Design review of the part built by this model. Coordinates are the model's own, in mm. A direction names the side the tool comes from. Coordinates: 2 decimals unless noted, no trailing zeros. Loops run counter-clockwise (first coordinate to the right, second up) from the corner with the lowest first, then second, coordinate; pieces in that order, holes last. Notation, with made-up numbers: (16.25, -19.5) -> (73.25, -19.5) arc R23 cw to (73.25, 5.5) -> close; hole circle Ø11 at (-10.75, -19). An arc over 180 degrees is marked (long way). Use a Markdown table: item, result. Add a question column.
Q1. Clearance check with flat-ended pins moving along their axes: pin 1 Ø0.9 at (y, z) = (22, 2) entering from -X; pin 2 Ø1.5 at (x, z) = (26.5, 2) entering from -Y; pin 3 Ø1.5 at (x, z) = (25.5, 2) entering from +Y. State where each tip first meets the part, or that it passes through.
Q2. For faces 1 (the face through (21.82, -22, 2)), 2 (the face through (-21.82, 22, 2)), 3 (the face through (21.82, 21, 2)), 4 (the face through (-27, -20, 2)), list the 3-axis set-ups (+Z, -Z, +X, -X, +Y, -Y) from which the entire face can be reached by the end or side of a thin tool; tool diameter is ignored.
Q3. Take a section at B-B on x = 22.5. Write out the cut boundary in (y, z).
Q4. Take a section at A-A on z = 1.2. Write out the cut boundary in (x, y).
Q5. For probe 1 along Y at (x, z) = (27, 2.25); probe 2 along X at (y, z) = (-21, 2.65), list the stretches that pass through material, from the lowest coordinate up.
Solid Edge part; units mm, degrees
sketch "Sketch1" plane through (0, 0, 0) normal (0, 0, 1) x (1, 0, 0)
  line L0 (-31.82, -23) -> (31.82, -23)
  line L1 (31.82, -23) -> (31.82, 23)
  line L2 (31.82, 23) -> (-31.82, 23)
  line L3 (-31.82, 23) -> (-31.82, -23)
  dimension "D1" = 31.82
  dimension "D2" = 31.82
extrude "Ajout_matière_1" add sketch "Sketch1" along normal blind 3
sketch "Sketch2" plane through (0, 0, 3) normal (0, 0, 1) x (1, 0, 0)
  line L0 (-31.82, 23) -> (-21.82, 23)
  line L1 (-21.82, 23) -> (-21.82, 20)
  line L2 (-21.82, 20) -> (-31.82, 20)
  line L3 (-31.82, 20) -> (-31.82, 23)
  dimension "D1" = 31.82
  dimension "D2" = 31.82
extrude "Cutout1" cut sketch "Sketch2" against normal through all
mirror "Mirror1" about plane through (0, 0, 0) normal (1, 0, 0) of "Cutout1"
mirror "Mirror2" about plane through (0, 0, 0) normal (0, -1, 0) of "Mirror1", "Cutout1"
properties material "Acier S235"
Answer list:
| question | item | result |
|---|---|---|
| 1 | pin 1 | x = -21.82 |
| 1 | pin 2 | y = -20 |
| 1 | pin 3 | y = 20 |
| 2 | face 1 | +Z, -Z, +X, -Y |
| 2 | face 2 | +Z, -Z, -X, +Y |
| 2 | face 3 | +Z, -Z, +X, +Y |
| 2 | face 4 | +Z, -Z, -X, -Y |
| 3 | outline | (-20, 0) -> (20, 0) -> (20, 3) -> (-20, 3) -> close |
| 4 | outline | (-31.82, -20) -> (-21.82, -20) -> (-21.82, -23) -> (21.82, -23) -> (21.82, -20) -> (31.82, -20) -> (31.82, 20) -> (21.82, 20) -> (21.82, 23) -> (-21.82, 23) -> (-21.82, 20) -> (-31.82, 20) -> close |
| 5 | probe 1 | -20 to 20 |
| 5 | probe 2 | -21.82 to 21.82 |
